Geometry: final body of the model. Coordinates: model frame, mm. Round coordinates to 2 decimals unless told otherwise and drop trailing zeros. Loops run counter-clockwise (first coordinate to the right, second up) from the corner with the lowest first, then second, coordinate; pieces in that order, holes last. Notation, with made-up numbers: (17, 51.25) - (36, 51.25) arc R22 ccw to (36, 75.25) - close; hole circle Ø11 at (80, 26.5). An arc over 180 degrees is marked (long way). Return JSON: item names as keys, results as strings. Group by question number.
1. Section A-A on z = 0.65. Count the separate pieces of the cut face and the enclosed holes in it, and give its area (3 significant figures).
2. First-contact query: pin 1 Ø1 at (x, y) = (11, 6.15) entering from +Z. Flat tip, straight axial feed; report the tip coordinate or a pass-through.
3. Draft query along X for faces 1 (the face through (-11.633, 4.168, 0.388)), 2 (the face through (-8.88, 10.6, 0.39)), 3 (the face through (0, 0, 0)). Return one class per face: +X half, -X half, draft (parallel to the pull), parting line (faces both ways), or undercut.
4. Section B-B on x = 9.75. Return loops of the section in (y, z).
5. Material intervals for probe 1 along X at (y, z) = (-8, 0.55); probe 2 along X at (y, z) = (-5.5, 0.15); probe 3 along Y at (x, z) = (7.25, 0.3), sorted ascending.
from build123d import *

# Parameters (mm, degrees)
CROQUIS1_R              = 0.635
SALIENTE_EXTRUIR1_DEPTH = 0.7874


with BuildPart() as part:
    # Croquis1 → Saliente-Extruir1 (new body)
    with BuildSketch(Plane.XY):
        Polygon((-5.6642, 13.8176), (-12.192, 7.2898), (-12.192, -13.8176), (12.192, -13.8176), (12.192, 7.2898), (5.6642, 13.8176), align=None)
        with Locations((-10.9982, -11.9126)):
            Circle(CROQUIS1_R, mode=Mode.SUBTRACT)
        with Locations((10.9982, -11.9126)):
            Circle(CROQUIS1_R, mode=Mode.SUBTRACT)
        with Locations((10.9982, -9.906)):
            Circle(CROQUIS1_R, mode=Mode.SUBTRACT)
        with Locations((10.9982, -7.8994)):
            Circle(CROQUIS1_R, mode=Mode.SUBTRACT)
        with Locations((10.9982, -5.8928)):
            Circle(CROQUIS1_R, mode=Mode.SUBTRACT)
        with Locations((10.9982, -3.8862)):
            Circle(CROQUIS1_R, mode=Mode.SUBTRACT)
        with Locations((10.9982, -1.8796)):
            Circle(CROQUIS1_R, mode=Mode.SUBTRACT)
        with Locations((10.9982, 0.127)):
            Circle(CROQUIS1_R, mode=Mode.SUBTRACT)
        with Locations((10.9982, 2.1336)):
            Circle(CROQUIS1_R, mode=Mode.SUBTRACT)
        with Locations((10.9982, 4.1402)):
            Circle(CROQUIS1_R, mode=Mode.SUBTRACT)
        with Locations((10.9982, 6.1468)):
            Circle(CROQUIS1_R, mode=Mode.SUBTRACT)
        with Locations((-10.9982, -9.906)):
            Circle(CROQUIS1_R, mode=Mode.SUBTRACT)
        with Locations((-10.9982, -7.8994)):
            Circle(CROQUIS1_R, mode=Mode.SUBTRACT)
        with Locations((-10.9982, -5.8928)):
            Circle(CROQUIS1_R, mode=Mode.SUBTRACT)
        with Locations((-10.9982, -3.8862)):
            Circle(CROQUIS1_R, mode=Mode.SUBTRACT)
        with Locations((-10.9982, -1.8796)):
            Circle(CROQUIS1_R, mode=Mode.SUBTRACT)
        with Locations((-10.9982, 0.127)):
            Circle(CROQUIS1_R, mode=Mode.SUBTRACT)
        with Locations((-10.9982, 2.1336)):
            Circle(CROQUIS1_R, mode=Mode.SUBTRACT)
        with Locations((-10.9982, 4.1402)):
            Circle(CROQUIS1_R, mode=Mode.SUBTRACT)
        with Locations((-10.9982, 6.1468)):
            Circle(CROQUIS1_R, mode=Mode.SUBTRACT)
    extrude(amount=SALIENTE_EXTRUIR1_DEPTH)


solid = part.part
Taken from the geometry:
{
 "1": {"separate pieces": "1", "enclosed holes": "20", "area": "606 mm2"},
 "2": {"pin 1": "through"},
 "3": {"face 1": "undercut", "face 2": "-X half", "face 3": "draft"},
 "4": {"outline": "(-13.82, 0) - (9.73, 0) - (9.73, 0.79) - (-13.82, 0.79) - close"},
 "5": {"probe 1": "-12.19 to -11.63, -10.37 to 10.37, 11.63 to 12.19", "probe 2": "-12.19 to -11.5, -10.5 to 10.5, 11.5 to 12.19", "probe 3": "-13.82 to 12.23"}
}
